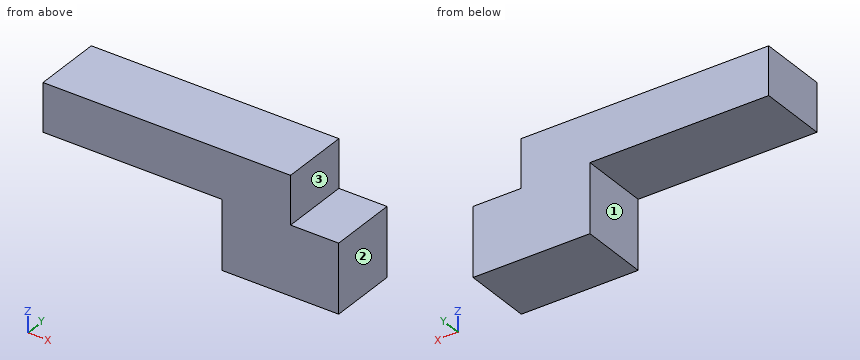
```python
from build123d import *

# Parameters (mm, degrees)
F0_W     = 91.44
F0_H     = 25.4
F1_DEPTH = 17.78
F2_W     = 25.4
F2_H     = 25.4
F3_DEPTH = 25.4
F4_W     = 25.4
F4_H     = 25.4
F5_DEPTH = 17.78


with BuildPart() as f1:
    # F0 (on Top) → F1 (new body)
    with BuildSketch(Plane.XY):
        with Locations((-14.985616, 46.367901)):
            Rectangle(F0_W, F0_H)
    extrude(amount=F1_DEPTH)

    # F2 (on face) → F3 (join)
    with BuildSketch(Plane(origin=(0, 0, 0), x_dir=(1, 0, 0), z_dir=(0, 0, -1))):
        with Locations((18.034384, -46.367901)):
            Rectangle(F2_W, F2_H)
    extrude(amount=F3_DEPTH)

    # F4 (on face) → F5 (join)
    with BuildSketch(Plane.YZ.offset(30.734384)):
        with Locations((46.367901, -12.7)):
            Rectangle(F4_W, F4_H)
    extrude(amount=F5_DEPTH)


solid = f1.part
```
Geometry check sheet. Reference: the model listing, model coordinates, mm. Face numbers are marked on the shaded views. A direction names the side the tool comes from. Coordinates: 2 decimals unless noted, no trailing zeros. Loops run counter-clockwise (first coordinate to the right, second up) from the corner with the lowest first, then second, coordinate; pieces in that order, holes last. Notation, with made-up numbers: (64.5, 46.5) - (97.5, 46.5) arc R34 cw to (97.5, 84.5) - close; hole circle Ø2 at (-30.75, -38.75). An arc over 180 degrees is marked (long way). One line per item, written item: value. Start each with the question number.
(1) Tool access check on the marked faces 1, 2 and 3. Record the directions out of +Z, -Z, +X, -X, +Y, -Y that give a thin tool (end or side, any length) a straight path to the whole face; none if there is none.
(2) Material ranges on line 1 (Z direction, x = -15, y = 38); line 2 (X direction, y = 38.5, z = 15); line 3 (X direction, y = 46.25, z = -13.5), recorded low to high. Write a range as [from, to].
(3) Cross-section at B-B on x = -19.5. Enter the section's corners in (y, z), plus the area to 3 significant figures.
(4) Cross-section at A-A on y = 36.5. Enter the section's corners in (x, z).
(5) Cross-section at C-C on z = 15. Enter the section's corners in (x, y), plus the area to 3 significant figures.
(6) Depth check by flat-ended pin: P1, Ø10, axis at x = -1, y = 56.5, coming from the -Z side; P2, Ø14, axis at y = 45.5, z = 8.5, coming from the +X side; P3, Ø12.5, axis at y = 49.5, z = -11.5, coming from the -X side. Enter the tip coordinate at first touch or a pass-through.
Results below:
1. face 1: -Z, -X, +Y, -Y
1. face 2: +Z, -Z, +X, +Y, -Y
1. face 3: +Z, +X, +Y, -Y
2. line 1: z = [0, 17.78]
2. line 2: x = [-60.71, 30.73]
2. line 3: x = [5.33, 48.51]
3. outline: (33.67, 0) - (59.07, 0) - (59.07, 17.78) - (33.67, 17.78) - close
3. area: 452 mm2
4. outline: (-60.71, 0) - (5.33, 0) - (5.33, -25.4) - (48.51, -25.4) - (48.51, 0) - (30.73, 0) - (30.73, 17.78) - (-60.71, 17.78) - close
5. outline: (-60.71, 33.67) - (30.73, 33.67) - (30.73, 59.07) - (-60.71, 59.07) - close
5. area: 2,320 mm2
6. P1: stops at z = 0
6. P2: stops at x = 30.73
6. P3: stops at x = 5.33
